Geometry check sheet. Reference: the model listing, model coordinates, mm. A direction names the side the tool comes from. Coordinates: 2 decimals unless noted, no trailing zeros. Write each loop counter-clockwise with the first axis right and the second up, starting at its lowest first coordinate (ties: lowest second). Pieces come first, ordered by that corner, then holes. Notation, with made-up numbers: (-17, -38.75) -> (42, -38.75) arc R15 ccw to (42, -15.75) -> close; hole circle Ø3 at (-19.5, -21.75). An arc over 180 degrees is marked (long way). One line per question, with ' | ' between items.
Autodesk Inventor part; units mm, degrees
ref_plane "YZ Plane" through (0, 0, 0) normal (1, 0, 0) x (0, 1, 0)
ref_plane "XZ Plane" through (0, 0, 0) normal (0, 1, 0) x (-1, 0, 0)
ref_plane "XY Plane" through (0, 0, 0) normal (0, 0, 1) x (1, 0, 0)
sketch "Sketch1" plane through (0, 0, 0) normal (0, 0, 1) x (1, 0, 0)
  circle A0 centre (0, 0) radius 5
  circle A1 centre (149.4, 0) radius 5
  circle A2 centre (85.7991, 21.6971) radius 5
  circle A3 centre (110.2989, -19.8991) radius 12.5
  arc A4 (154.885, -2.4321) -> (154.9491, -2.282) centre (149.4, 0) ccw
  line L0 (-1.9594, 5.6711) -> (-0.9713, 5.9209)
  line L1 (94.051, 25.713) -> (120.8026, 18.6971)
  arc A5 (131.5219, 14.0064) -> (120.0887, 18.8843) centre (110.2989, -19.8991) ccw
  line L2 (0, 0) -> (4.8474, 1.2258)
  line L3 (80.8741, 20.8344) -> (85.7991, 21.6971)
  arc A6 (125.9738, -56.7) -> (149.4311, -28.1861) centre (110.2989, -19.8991) ccw
  line L4 (80.7723, -79.2884) -> (129.3991, -55.0443)
  line L5 (-0.8206, -9.3961) -> (37.9799, -67.1663)
  arc A7 (90.3858, 23.6876) -> (86.8225, 21.8764) centre (110.2989, -19.8991) ccw
  arc A8 (33.9775, -61.2072) -> (80.7723, -79.2884) centre (68.0362, -42.6558) ccw
  line L6 (131.5219, 14.0064) -> (145.3135, 8.2114)
  line L7 (150.7621, 5.922) -> (151.3594, 5.6711)
  line L8 (154.928, -2.2287) -> (154.885, -2.4321)
  line L9 (153.6652, -8.1921) -> (149.4311, -28.1861)
  arc A9 (154.9491, -2.282) -> (154.3356, -0.8001) centre (110.2989, -19.8991) ccw
  arc A10 (151.6581, 4.4611) -> (150.7621, 5.922) centre (110.2989, -19.8991) ccw
  arc A11 (-0.9713, 5.9209) -> (-1.9594, 5.6711) centre (0, 0) ccw
  arc A12 (-4.6746, 3.7614) -> (-4.9033, 3.458) centre (55.8634, -42.1071) ccw
  arc A13 (-4.6746, 3.7614) -> (-4.9033, 3.458) centre (0, 0) ccw
  arc A14 (50.3563, 33.7779) -> (18.6552, 24.2587) centre (44.1835, -3.2106) ccw
  arc A15 (80.9569, 29.5804) -> (51.4686, 33.7181) centre (55.8634, -42.1071) ccw
  arc A16 (17.7599, 23.5959) -> (-0.1619, 9.1758) centre (55.8634, -42.1071) ccw
  arc A17 (17.7599, 23.5959) -> (18.6552, 24.2587) centre (15.2515, 27.9212) ccw
  arc A18 (50.3563, 33.7779) -> (51.4686, 33.7181) centre (51.1793, 38.7097) ccw
  arc A19 (91.6578, 27.1447) -> (83.8358, 29.4525) centre (85.7991, 21.6971) ccw
  arc A20 (155.0349, -5.6787) -> (148.0771, 7.8899) centre (149.4, 0) ccw
  arc A21 (155.0349, -5.6787) -> (153.6652, -8.1921) centre (158.5567, -9.2279) ccw
  arc A22 (145.3135, 8.2114) -> (148.0771, 7.8899) centre (147.2503, 12.821) ccw
  arc A23 (80.9569, 29.5804) -> (83.8358, 29.4525) centre (82.6088, 34.2996) ccw
  arc A24 (91.6578, 27.1447) -> (94.051, 25.713) centre (95.3194, 30.5494) ccw
  arc A25 (-2.6216, 7.5583) -> (-3.3151, -7.2808) centre (0, 0) ccw
  arc A26 (-0.8206, -9.3961) -> (-3.3151, -7.2808) centre (-5.8014, -12.7414) ccw
  arc A27 (-2.6216, 7.5583) -> (-0.1619, 9.1758) centre (-4.5877, 13.227) ccw
  point P0 (90.8386, 26.5555)
  point P1 (111.3369, -59.8857)
  point P2 (-4.37, -4.1113)
  point P3 (148.3758, 6.9247)
  point P4 (154.3524, -4.9471)
  point P5 (92.4582, 26.1307)
  point P6 (146.8277, 7.5752)
  point P7 (154.0164, -6.5337)
  point P8 (-1.9144, -7.7676)
  dimension "d3" = 10
  dimension "d5" = 10
  dimension "d15" = 10
  dimension "d18" = 25
  dimension "d20" = 12
  dimension "d104" = 75
  dimension "d105" = 5
  dimension "d112" = 16
  dimension "d113" = 16
  dimension "d114" = 5
  dimension "d115" = 16
  dimension "d116" = 6
extrude "Extrusion2" add sketch "Sketch1" along normal blind 28 contours A9 A4 L8 | L1 A5 L6 A22 A20 A21 L9 A6 L4 A8 L5 A26 A25 A27 A16 A17 A14 A18 A15 A23 A19 A24 | A12 A13
sketch "Sketch13" plane through (0, 0, 28) normal (0, 0, 1) x (1, 0, 0)
  arc A0 (105.7808, -55.6145) -> (122.4659, 13.9825) centre (110.2989, -19.8991) ccw
  line L0 (32.2727, -40.0871) -> (32.3131, -38.891)
  circle A1 centre (85.7991, 21.6971) radius 5
  arc A2 (122.3009, 14.0385) -> (99.574, 19.2733) centre (79.666, -119.1093) ccw
  arc A3 (75.8397, 22.5968) -> (71.8542, 27.9468) centre (70.8599, 23.0467) ccw
  arc A4 (99.574, 19.2733) -> (94.5077, 16.7819) centre (98.8621, 14.3243) ccw
  arc A5 (105.7808, -55.6145) -> (100.6423, -58.4183) centre (105.1533, -60.575) ccw
  arc A6 (32.3131, -38.891) -> (31.6808, -35.0382) centre (22.3188, -38.553) ccw
  arc A7 (71.8542, 27.9468) -> (53.5851, 30.0522) centre (55.1602, -36.5967) ccw
  arc A8 (45.4586, 29.4346) -> (46.2799, 29.4767) centre (45.6139, 34.4322) ccw
  arc A9 (122.4659, 13.9825) -> (122.3009, 14.0385) centre (120.7761, 9.2767) ccw
  arc A10 (32.2727, -40.0871) -> (100.6423, -58.4183) centre (68.36, -42.1569) ccw
  arc A11 (75.8397, 22.5968) -> (94.5077, 16.7819) centre (85.7991, 21.6971) ccw
  arc A12 (21.1272, 20.7085) -> (21.4488, 20.9624) centre (18.1914, 24.7558) ccw
  arc A13 (52.3778, 30.1709) -> (7.5869, -5.4513) centre (44.3656, -5.7255) ccw
  arc A14 (7.6133, -6.0028) -> (28.5671, -32.0476) centre (38.2081, -2.8397) ccw
  arc A15 (26.215, -29.3432) -> (26.5512, -29.4928) centre (38.2081, -2.8397) ccw
  arc A16 (52.3778, 30.1709) -> (53.5851, 30.0522) centre (53.467, 35.0508) ccw
  arc A17 (7.5869, -5.4513) -> (7.6133, -6.0028) centre (12.5868, -5.4886) ccw
  arc A18 (31.6808, -35.0382) -> (28.5671, -32.0476) centre (26.9998, -36.7956) ccw
  point P0 (0, 0)
  point P1 (44.2138, -2.45)
  point P2 (68.1634, -42.8903)
  point P3 (32.5739, -31.1818)
  dimension "d97" = 5
  dimension "d99" = 10
  dimension "d106" = 5
  dimension "d107" = 5
  dimension "d108" = 5
  dimension "d111" = 5
extrude "Extrusion18" cut sketch "Sketch13" against normal blind 30 contours A5 A10 L0 A6 A18 A14 A17 A13 A16 A7 A3 A11 A4 A2 A9 A0
properties part number "body gauche"
1. Cross-section at A-A on y = -2.5. Record the boundary of the cut face in (x, z).
Worked answers:
outline: (-7.6, 0) -> (-4.33, 0) -> (-4.33, 28) -> (-7.6, 28) -> close; (4.33, 0) -> (7.73, 0) -> (7.73, 28) -> (4.33, 28) -> close; (141.82, 0) -> (145.07, 0) -> (145.07, 28) -> (141.82, 28) -> close; (153.73, 0) -> (157, 0) -> (157, 28) -> (153.73, 28) -> close
2. Tool access check on faces 1 (the face through (32.19, -36.96, 14.2)), 2 (the face through (80, 15, 28)). Record the directions out of +Z, -Z, +X, -X, +Y, -Y that give a thin tool (end or side, any length) a straight path to the whole face; none if there is none.
Worked answers:
face 1: +Z, -Z | face 2: +Z, +X, -X, +Y, -Y
3. Cross-section at D-D on z = 14.25. Give the number of separate pieces and of enclosed holes in the cut face, and give its area (3 significant figures).
Worked answers:
separate pieces: 1 | enclosed holes: 5 | area: 2,250 mm²
4. Cross-section at C-C on y = -52. Record the boundary of the cut face in (x, z), and give its area (3 significant figures).
Worked answers:
outline: (27.79, 0) -> (33.58, 0) -> (33.58, 28) -> (27.79, 28) -> close; (126.59, 0) -> (134.16, 0) -> (134.16, 28) -> (126.59, 28) -> close | area: 374 mm²
5. Cross-section at B-B on x = 44. Record the boundary of the cut face in (y, z), and give its area (3 significant figures).
Worked answers:
outline: (-73.09, 0) -> (-68.86, 0) -> (-68.86, 28) -> (-73.09, 28) -> close; (31.05, 0) -> (34.29, 0) -> (34.29, 28) -> (31.05, 28) -> close | area: 209 mm²
6. Mould release check, pull along Y, two halves, no side actions. Record for faces 3 (the face through (88.005, 29.387, 13.804)), 4 (the face through (-1.08, 4.88, 13.8)), 5 (the face through (57.79, -80.06, 13.8)): released by +Y, released by -Y, zero draft, split by the parting line, or undercut.
Worked answers:
face 3: released by +Y | face 4: undercut | face 5: released by -Y
7. Go/stop test with flat-tipped pins: P1, Ø2, axis at x = 25.5, z = 3.5, coming from the +Y side; P2, Ø4, axis at x = 59, z = 22.5, coming from the -Y side; P3, Ø4, axis at x = 104, z = 19.5, coming from the -Y side; P4, Ø11.5, axis at x = 0, y = 0, coming from the -Z side. Record where each tip stops, or that it passes through.
Worked answers:
P1: y = 29.86 | P2: y = -80.8 | P3: y = -68.7 | P4: z = 0
8. Material ranges on line 1 (Y direction, x = 85.5, z = 15.5); line 2 (Y direction, x = 71, z = 12.75); line 3 (Y direction, x = 110, z = 18), recorded low to high. Write a range as from..to.
Worked answers:
line 1: -76.93..-73.98, 11.7..16.71, 26.69..29.69 | line 2: -81.33..-78.21, 28.16..32.32 | line 3: -64.72..-55.9, 17.37..21.53
